```python
from build123d import *

# Parameters (mm, degrees)
SKETCH_1_R            = 2.75
EXTRUDE_248_DEPTH     = 3
CUT_EXTRUDE_378_DEPTH = 1.3
SKETCH_3_R            = 1.5
EXTRUDE_479_DEPTH     = 22


with BuildPart() as part:
    # 草图1 → Extrude 248 (new body)
    with BuildSketch(Plane(origin=(0, 0, 0), x_dir=(1, 0, 0), z_dir=(0, 1, 0))):
        Circle(SKETCH_1_R)
    extrude(amount=EXTRUDE_248_DEPTH)

    # 草图2 → Cut-Extrude 378 (cut)
    with BuildSketch(Plane(origin=(0, 3, 0), x_dir=(1, 0, 0), z_dir=(0, 1, 0))):
        Polygon((1.443375673, 0), (0.721687836, 1.25), (-0.721687836, 1.25), (-1.443375673, 0), (-0.721687836, -1.25), (0.721687836, -1.25), align=None)
    extrude(amount=-CUT_EXTRUDE_378_DEPTH, mode=Mode.SUBTRACT)

    # 草图3 → Extrude 479 (add)
    with BuildSketch(Plane.XZ):
        Circle(SKETCH_3_R)
    extrude(amount=EXTRUDE_479_DEPTH)


solid = part.part
```
Here's how the part is built. I have some questions about the finished solid (model axes, mm). A direction names the side the tool comes from. Coordinates: 2 decimals unless noted, no trailing zeros. Order: outer loops, then holes, each group sorted by start corner. A loop starts at its lowest first (then second) coordinate and runs counter-clockwise, first axis right, second up. Notation, with made-up numbers: (88.25, 6.5) -> (114.25, 6.5) arc R21 cw to (114.25, 15.5) -> close; hole circle Ø2 at (-4.5, 69). An arc over 180 degrees is marked (long way). Return JSON: item names as keys, results as strings.
1) Thinking about a two-plate mould opening in X: for faces 4 (the flat face through (-1.08, 2.36, -0.63)), 5 (the cylindrical face through (-1.5, -10.85, 0.07)), 6 (the flat face through (0, -22, 0)), which applies, +X half, -X half, draft (parallel to the pull), parting line (faces both ways), or undercut?
Conclusion:
{"face 4": "undercut", "face 5": "parting line", "face 6": "draft"}
2) If we section it at A-A on x = 0: List the corners of the cut face in (y, z) for me, plus the area to 4 significant figures.
Conclusion:
{"outline": "(-22, -1.5) -> (0, -1.5) -> (0, -2.75) -> (3, -2.75) -> (3, -1.25) -> (1.7, -1.25) -> (1.7, 1.25) -> (3, 1.25) -> (3, 2.75) -> (0, 2.75) -> (0, 1.5) -> (-22, 1.5) -> close", "area": "79.25 mm²"}
3) If we section it at C-C on y = -3.25: List the corners of the cut face in (x, z) for me.
Conclusion:
{"outline": "circle Ø3 at (0, 0)"}
4) On a 3-axis mill with a long thin cutter (end or side, diameter ignored), from which of +Z, -Z, +X, -X, +Y, -Y can I reach the whole of each face in a straight line? I mean faces 1 (the flat face through (1.2, 0, 1.2)), 2 (the flat face through (-1.3, 3, 0.6)), 3 (the flat face through (0, 1.7, 0)). Say none if no direction works.
Conclusion:
{"face 1": "-Y", "face 2": "+Z, -Z, +X, -X, +Y", "face 3": "+Y"}
5) If I drill on probe 1 along Y at (x, z) = (0.85, -1.35); probe 2 along Z at (x, y) = (-0.1, -8); probe 3 along Y at (x, z) = (1, 0.5), over which ranges is the centre line in solid material (lowest first)?
Conclusion:
{"probe 1": "y = 0 to 3", "probe 2": "z = -1.5 to 1.5", "probe 3": "y = -22 to 1.7"}
6) If we section it at B-B on z = 0.25: List the corners of the cut face in (x, y) for me, plus the area to 3 significant figures.
Conclusion:
{"outline": "(-2.74, 0) -> (-1.48, 0) -> (-1.48, -22) -> (1.48, -22) -> (1.48, 0) -> (2.74, 0) -> (2.74, 3) -> (1.3, 3) -> (1.3, 1.7) -> (-1.3, 1.7) -> (-1.3, 3) -> (-2.74, 3) -> close", "area": "78.1 mm²"}
7) If we section it at D-D on z = -2.35: List the corners of the cut face in (x, y) for me.
Conclusion:
{"outline": "(-1.43, 0) -> (1.43, 0) -> (1.43, 3) -> (-1.43, 3) -> close"}
